Geometry: final body of the model. Coordinates: model frame, mm. A direction names the side the tool comes from. Give positions to 0.01 mm unless a question says otherwise; leave off trailing zeros. Write each loop counter-clockwise with the first axis right and the second up, starting at its lowest first coordinate (ties: lowest second). Pieces come first, ordered by that corner, then holes.
Q1. Pin query (flat end, axial travel): pin 1 Ø1 at (x, y) = (-2.5, 49) entering from -Z; pin 2 Ø1.6 at (x, z) = (-1.5, 4) entering from -Y; pin 3 Ø2.5 at (x, y) = (-1, 14.5) entering from +Z. Return the tip coordinate at first contact, or that it passes through.
Q2. Mould query, pull axis X, two halves, no side actions, for faces 1 (the cylindrical face through (1.5, 64.09, 4.77)), 2 (the flat face through (2, 8, -2)), 3 (the cylindrical face through (-0.54, 7.56, 0.56)). Classes: +X half, -X half, draft (parallel to the pull), parting line (faces both ways), or undercut.
Q3. Section C-C (z = 0). Return the cut outline in (x, y).
Q4. Section D-D (y = 52.5). Return the cut outline in (x, z).
Q5. Line query: line 1 (Z direction, x = -0.25, y = 38.5); line 2 (Y direction, x = 0.75, z = -3.25); line 3 (Y direction, x = -2.25, z = 2). Output: solid intervals per line, ascending.
Q6. Reachability of faces 4 (the flat face through (0, 130, 0)), 5 (the flat face through (0, 20, -3)), 6 (the flat face through (-3, 10, 3.059)) from +Z, -Z, +X, -X, +Y, -Y: full face, straight path, thin tool, end or side. Return the list, or none.
Q7. Section A-A (y = 10). Return the cut outline in (x, z), plus the area to 3 significant figures.
Q8. Section B-B (x = 0). Return the cut outline in (y, z).
from build123d import *

# Parameters (mm, degrees)
ESQUISSE1_R             = 5
BOSS_EXTRU_1_DEPTH      = 130
ENL_V_MAT_EXTRU_2_DEPTH = 20
ENL_V_MAT_EXTRU_3_DEPTH = 20
ESQUISSE4_R             = 2.5
ENL_V_MAT_EXTRU_4_DEPTH = 60


with BuildPart() as part:
    # Esquisse1 → Boss.-Extru.1 (new body)
    with BuildSketch(Plane(origin=(0, 0, 0), x_dir=(1, 0, 0), z_dir=(0, 1, 0))):
        with Locations(Location((0, 0, 0), (0, 0, 270))):
            Circle(ESQUISSE1_R)
    extrude(amount=BOSS_EXTRU_1_DEPTH)

    # Esquisse2 → Enlèv. mat.-Extru.2 (cut)
    with BuildSketch(Plane(origin=(0, 0, 0), x_dir=(-1, 0, 0), z_dir=(0, -1, 0))):
        with BuildLine():
            Line((-4.582575695, 2), (4.582575695, 2))
            ThreePointArc((4.582575695, 2), (4.582464701, 2.0002543), (4.582353692, 2.000508595))
            ThreePointArc((4.582353692, 2.000508595), (-0.000277468, 4.999999992), (-4.582575695, 2))
        make_face()
    extrude(amount=-ENL_V_MAT_EXTRU_2_DEPTH, mode=Mode.SUBTRACT)

    # Esquisse3 → Enlèv. mat.-Extru.3 (cut)
    with BuildSketch(Plane.XZ):
        with BuildLine():
            ThreePointArc((3.95513796, 3.058902371), (0, 5), (-3.95513796, 3.058902371))
            Line((-3.95513796, 3.058902371), (3.95513796, 3.058902371))
        make_face()
    extrude(amount=-ENL_V_MAT_EXTRU_3_DEPTH, mode=Mode.SUBTRACT)

    # Esquisse4 → Enlèv. mat.-Extru.4 (cut)
    with BuildSketch(Plane.XY.offset(3.058902371)):
        with Locations((0.00513796, 10)):
            Circle(ESQUISSE4_R)
    extrude(amount=-ENL_V_MAT_EXTRU_4_DEPTH, mode=Mode.SUBTRACT)


solid = part.part
Computed:
1. pin 1: stops at z = -4.58
1. pin 2: stops at y = 20
1. pin 3: stops at z = 3.06
2. face 1: parting line
2. face 2: draft
2. face 3: undercut
3. outline: (-5, 0) - (5, 0) - (5, 130) - (-5, 130) - close; hole circle Ø5 at (0.01, 10)
4. outline: circle Ø10 at (0, 0)
5. line 1: z = -4.99 to 4.99
5. line 2: y = 20 to 130
5. line 3: y = 0 to 8.92, 11.08 to 130
6. face 4: +Z, -Z, +X, -X, +Y
6. face 5: -Z, +X, -X, -Y
6. face 6: +Z, +X, -X, -Y
7. outline: (-4.58, -2) - (-2.49, -2) - (-2.49, 3.06) - (-3.96, 3.06) arc R5 ccw to start; (2.51, -2) - (4.58, -2) arc R5 ccw to (3.96, 3.06) - (2.51, 3.06) - close
7. area: 22.7 mm2
8. outline: (0, -2) - (7.5, -2) - (7.5, 3.06) - (0, 3.06) - close; (12.5, -2) - (20, -2) - (20, -5) - (130, -5) - (130, 5) - (20, 5) - (20, 3.06) - (12.5, 3.06) - close
